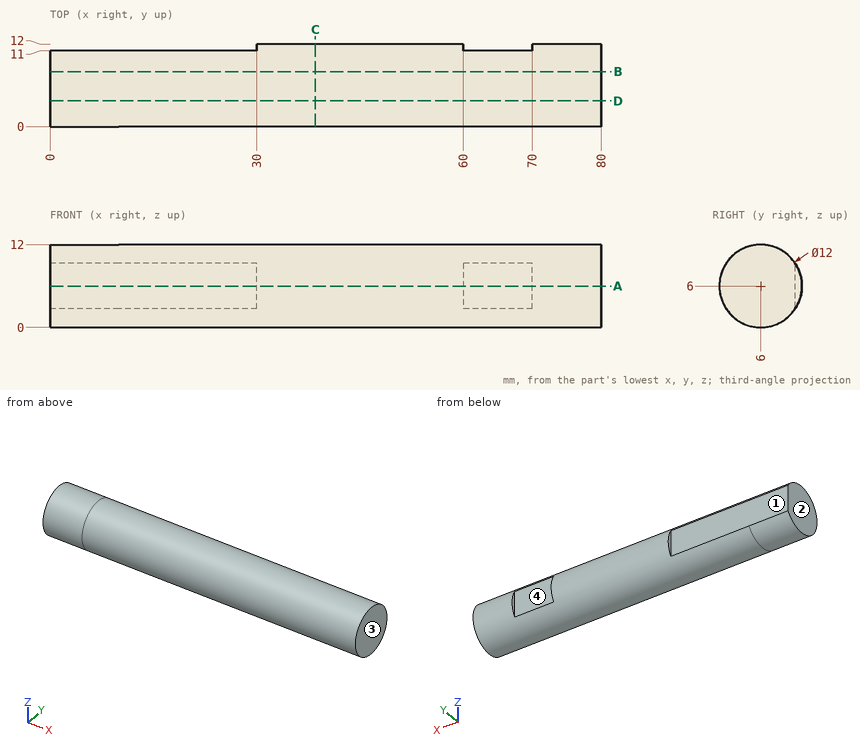
Print and shaded views of the part. All mm, measured from the part's lowest x, y and z. Coordinates: 2 decimals unless noted, no trailing zeros. Order: outer loops, then holes, each group sorted by start corner. A loop starts at its lowest first (then second) coordinate and runs counter-clockwise, first axis right, second up. Notation, with made-up numbers: M 46.25,-32.5 L 61.25,-32.5 A23 ccw 61.25,3.5 Z; hole C 88,89 d3. An arc over 180 degrees is marked long. One line per question, with ' | ' between items. Start each with the question number.
Q1. Probe L1, parallel to Z at x = 46, y = 1; L2, parallel to Z at x = 70, y = 1.5. List the from-to ranges inside material, lowest first. Write a range as from..to.
Q2. Two-plate mould, pull along X, no slides. Class the marked faces 1, 2, 3 and 4: +X half, -X half, draft (parallel to the pull), parting line (faces both ways), or undercut.
Q3. Saw through at D-D (y = 3.75). List the corners of the cut face in (x, z).
Q4. Saw through at C-C (x = 38.5). List the corners of the cut face in (y, z).
Q5. Saw through at B-B (y = 8). List the corners of the cut face in (x, z), then the cut area to 3 significant figures.
Q6. Saw through at A-A (z = 6). List the corners of the cut face in (x, y), then the cut area to 3 significant figures.
Q7. Flat gauge pins, fed straight in: pin 1 Ø1 at (y, z) = (8, 2.5) entering from -X; pin 2 Ø1.5 at (x, y) = (18, 10.5) entering from -Z; pin 3 Ø0.8 at (y, z) = (11.5, 7.5) entering from -X; pin 4 Ø2 at (x, z) = (59, 1) entering from +Y. Where does each tip first touch, or does it go through?
Check values:
1) L1: z = 2.68..9.32 | L2: z = 2.03..9.97
2) face 1: draft | face 2: -X half | face 3: +X half | face 4: undercut
3) outline: M 0,0.44 L 80,0.44 L 80,11.56 L 0,11.56 Z
4) outline: C 6,6 d12
5) outline: M 0,0.34 L 80,0.34 L 80,11.66 L 0,11.66 Z | area: 905 mm2
6) outline: M 0,0 L 80,0 L 80,12 L 70,12 L 70,11 L 60,11 L 60,12 L 30,12 L 30,11 L 0,11 Z | area: 920 mm2
7) pin 1: stops at x = 0 | pin 2: stops at z = 1.32 | pin 3: stops at x = 30 | pin 4: stops at y = 10.47
